The listing builds one solid part. Answer for the finished solid, in the listing's coordinates (mm). A direction names the side the tool comes from. Give positions to 0.01 mm unless a question says otherwise; leave off trailing zeros. Write each loop counter-clockwise with the first axis right and the second up, starting at its lowest first coordinate (ties: lowest second). Pieces come first, ordered by that corner, then holes. Notation, with made-up numbers: (59.25, 37.5) - (118.25, 37.5) arc R17 cw to (118.25, 61.5) - close; hole circle Ø7 at (42.25, -22.5). An arc over 180 degrees is marked (long way). Return JSON: item names as keys, results as strings.
from build123d import *

# Parameters (mm, degrees)
CROQUIS1_W              = 5.6
CROQUIS1_H              = 2.6
SALIENTE_EXTRUIR1_DEPTH = 17
CROQUIS2_W              = 1.5
CROQUIS2_H              = 1.5
CORTAR_EXTRUIR1_DEPTH   = 3
REDONDEO1_R             = 0.25


with BuildPart() as part:
    # Croquis1 → Saliente-Extruir1 (new body)
    with BuildSketch(Plane.YZ):
        Rectangle(CROQUIS1_W, CROQUIS1_H)
    extrude(amount=SALIENTE_EXTRUIR1_DEPTH)

    # Croquis2 → Cortar-Extruir1 (cut)
    with BuildSketch(Plane.YZ.offset(17)):
        with Locations((1.375, 0)):
            Rectangle(CROQUIS2_W, CROQUIS2_H)
        with Locations((-1.375, 0)):
            Rectangle(CROQUIS2_W, CROQUIS2_H)
    extrude(amount=-CORTAR_EXTRUIR1_DEPTH, mode=Mode.SUBTRACT)

    # Redondeo1
    redondeo1_edges = [part.edges().sort_by_distance(p)[0] for p in [
        (17, -2.8, 0),
        (17, 0, -1.3),
        (17, 2.8, 0),
        (0, 0, -1.3),
        (0, -2.8, 0),
        (0, 0, 1.3),
        (0, 2.8, 0),
        (8.5, 2.8, -1.3),
        (8.5, -2.8, -1.3),
        (8.5, -2.8, 1.3),
        (8.5, 2.8, 1.3),
        (17, 0, 1.3),
    ]]
    fillet(redondeo1_edges, radius=REDONDEO1_R)


solid = part.part
Item 1: For faces 4 (the face through (8, 0, 1.3)), 5 (the face through (16, -1, -0.75)), determine the directions among +Z, -Z, +X, -X, +Y, -Y from which every point of the face is accessible in a straight line to the end or side of a thin tool.
Answer below:
{"face 4": "+Z, +X, -X, +Y, -Y", "face 5": "+X"}
Item 2: The mould has two halves that part along Y. Classify faces 1 (the face through (16, 1, -0.75)), 2 (the face through (8, 2.8, 0)), 3 (the face through (0, 0, 0)): +Y half, -Y half, draft (parallel to the pull), parting line (faces both ways), or undercut.
Answer below:
{"face 1": "undercut", "face 2": "+Y half", "face 3": "draft"}
Item 3: A flat-ended cylindrical pin translates along its axis: P1, Ø0.8, axis at y = -1.5, z = 0, coming from the +X side. Find the tip coordinate at first contact, or state that the pin passes through.
Answer below:
{"P1": "stops at x = 14"}
Item 4: A cutting plane is placed at A-A on z = 0.5. Determine the outline of the cut face in (x, y) (3 decimals).
Answer below:
{"outline": "(0, -2.55) arc R0.25 ccw to (0.25, -2.8) - (16.75, -2.8) arc R0.25 ccw to (17, -2.55) - (17, -2.125) - (14, -2.125) - (14, -0.625) - (17, -0.625) - (17, 0.625) - (14, 0.625) - (14, 2.125) - (17, 2.125) - (17, 2.55) arc R0.25 ccw to (16.75, 2.8) - (0.25, 2.8) arc R0.25 ccw to (0, 2.55) - close"}
Item 5: A cutting plane is placed at B-B on y = -1.55. Determine the outline of the cut face in (x, z).
Answer below:
{"outline": "(0, -1.05) arc R0.25 ccw to (0.25, -1.3) - (16.75, -1.3) arc R0.25 ccw to (17, -1.05) - (17, -0.75) - (14, -0.75) - (14, 0.75) - (17, 0.75) - (17, 1.05) arc R0.25 ccw to (16.75, 1.3) - (0.25, 1.3) arc R0.25 ccw to (0, 1.05) - close"}
Item 6: Consider L1, parallel to Z at x = 14.75, y = 1.45; L2, parallel to X at y = -1.25, z = 1.15; L3, parallel to X at y = 1.2, z = 0.4. Determine where each line is inside the solid, lowest interval first.
Answer below:
{"L1": "z = -1.3 to -0.75, 0.75 to 1.3", "L2": "x = 0.02 to 16.98", "L3": "x = 0 to 14"}
